Part model, mm, in its own coordinate system. Face numbers are marked on the shaded views. A direction names the side the tool comes from. Coordinates: 2 decimals unless noted, no trailing zeros. Loops run counter-clockwise (first coordinate to the right, second up) from the corner with the lowest first, then second, coordinate; pieces in that order, holes last. Notation, with made-up numbers: (-33, 67.5) - (23, 67.5) arc R19 cw to (23, 92.5) - close; hole circle Ø7 at (42.5, -9.5). An arc over 180 degrees is marked (long way). Use a Markdown table: item, result. Add a question column.
1. Drop flat-ended pins along their axis: pin 1 (5.5 mm diameter, centred on y = 8.5, z = -5, fed in from +X); pin 2 (9 mm diameter, centred on y = 9.5, z = 9.5, fed in from -X); pin 3 (4.5 mm diameter, centred on y = 19.3, z = 19.3, fed in from +X). Give the stop position or say it passes through.
2. 3-axis set-ups, long thin cutter, end or side, ignore diameter. For the marked faces 5 and 6: which of +Z, -Z, +X, -X, +Y, -Y reach the whole face in a straight line?
3. Band-saw the part on B-B, the plane z = 13.5. Give the cut face in (x, y), plus the area to 3 significant figures.
4. Band-saw the part on D-D, the plane y = -16. Give the cut face in (x, z), plus the area to 3 significant figures.
5. Wall check: probe 1 along Z at (x, y) = (6.5, -19.3) (3 decimals); probe 2 along Y at (x, z) = (33.5, -7); probe 3 along Y at (x, z) = (33, 13.5). Give the ranges that are in metal, low to high. Write a range as [from, to].
6. Pull direction Z, two halves, no side cores. Call the marked faces 1, 2, 3 and 4: pulls with the +Z half, pulls with the -Z half, needs draft (parallel to the pull), parting line crosses it, or undercut.
7. Band-saw the part on C-C, the plane y = -8. Give the cut face in (x, z), plus the area to 3 significant figures.
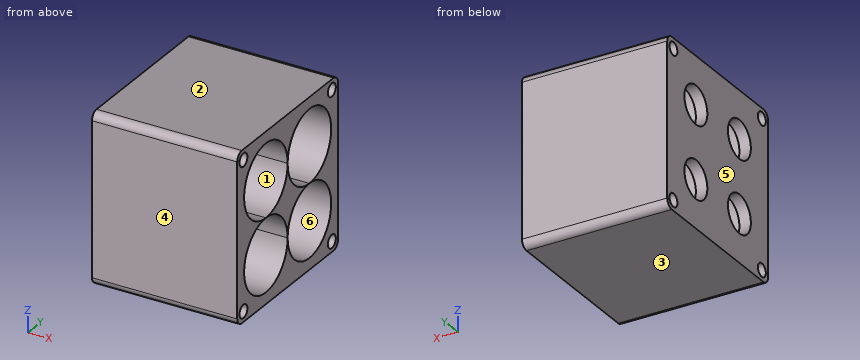
Autodesk Inventor part; units mm, degrees
ref_plane "YZ Plane" through (0, 0, 0) normal (1, 0, 0) x (0, 1, 0)
ref_plane "XZ Plane" through (0, 0, 0) normal (0, 1, 0) x (-1, 0, 0)
ref_plane "XY Plane" through (0, 0, 0) normal (0, 0, 1) x (1, 0, 0)
sketch "Sketch1" plane through (0, 0, 0) normal (1, 0, 0) x (0, 1, 0)
  line L0 (-22, -22) -> (22, -22)
  line L1 (22, -22) -> (22, 22)
  line L2 (22, 22) -> (-22, 22)
  line L3 (-22, 22) -> (-22, -22)
  line L4 (-22, -22) -> (22, 22) construction
  line L5 (22, -22) -> (-22, 22) construction
  line L6 (-19.3, -19.3) -> (19.3, -19.3)
  line L7 (19.3, -19.3) -> (19.3, 19.3)
  line L8 (19.3, 19.3) -> (-19.3, 19.3)
  line L9 (-19.3, 19.3) -> (-19.3, -19.3)
  line L10 (-19.3, -19.3) -> (19.3, 19.3) construction
  line L11 (19.3, -19.3) -> (-19.3, 19.3) construction
  circle A0 centre (19.3, 19.3) radius 1.725
  circle A1 centre (19.3, -19.3) radius 1.725
  circle A2 centre (-19.3, -19.3) radius 1.725
  circle A3 centre (-19.3, 19.3) radius 1.725
  circle A4 centre (9.5, 9.5) radius 9.5
  circle A5 centre (9.5, -9.5) radius 9.5
  circle A6 centre (-9.5, -9.5) radius 9.5
  circle A7 centre (-9.5, 9.5) radius 9.5
  point P0 (0, 0)
  point P1 (0, 0)
  point P2 (0, 0)
  point P3 (-9.5, 0)
  point P4 (0, 9.5)
  point P5 (9.5, 0)
  point P6 (0, -9.5)
  dimension "d4" = 44
  dimension "d5" = 44
  dimension "d6" = 38.6
  dimension "d7" = 3.45
  dimension "d8" = 3.45
  dimension "d9" = 3.45
  dimension "d10" = 3.45
  dimension "d24" = 19
  dimension "d25" = 19
  dimension "d26" = 19
  dimension "d27" = 19
extrude "Extrusion1" add sketch "Sketch1" along normal blind 35 contours L3 L2 L1 L0 | A2 L9 A3 L8 A0 L7 A1 L6 | A4 A5 A6 A7
fillet "Fillet1" radius 2 4 edges at (17.5, -22, 22) (17.5, -22, -22) (17.5, 22, 22) (17.5, 22, -22)
sketch "Sketch3" plane through (0, 0, 0) normal (-1, 0, 0) x (0, 0, 1)
  circle A0 centre (19.3, 19.3) radius 1.725
  arc A1 (0, -9.5) -> (9.5, 0) centre (9.5, -9.5) ccw
  arc A2 (-9.5, 0) -> (0, -9.5) centre (-9.5, -9.5) ccw
  arc A3 (0, 9.5) -> (-9.5, 0) centre (-9.5, 9.5) ccw
  arc A4 (9.5, 0) -> (0, 9.5) centre (9.5, 9.5) ccw
  circle A5 centre (-19.3, 19.3) radius 1.725
  circle A6 centre (-19.3, -19.3) radius 1.725
  circle A7 centre (19.3, -19.3) radius 1.725
  arc A8 (22, 20) -> (20, 22) centre (20, 20) ccw
  line L0 (-20, 22) -> (20, 22)
  line L1 (-22, -20) -> (-22, 20)
  arc A9 (-22, -20) -> (-20, -22) centre (-20, -20) ccw
  line L2 (20, -22) -> (-20, -22)
  arc A10 (20, -22) -> (22, -20) centre (20, -20) ccw
  line L3 (22, 20) -> (22, -20)
  circle A11 centre (9.5, -9.5) radius 5
  circle A12 centre (-9.5, -9.5) radius 5
  circle A13 centre (-9.5, 9.5) radius 5
  circle A14 centre (9.5, 9.5) radius 5
  arc A15 (-20, 22) -> (-22, 20) centre (-20, 20) ccw
  point P0 (0, 0)
  dimension "d28" = 10
  dimension "d29" = 10
  dimension "d30" = 10
  dimension "d31" = 10
extrude "Extrusion3" add sketch "Sketch3" along normal blind 3 contours A2 A3 A4 A1 | L3 A10 L2 A9 L1 A15 L0 A8
properties part number "BatteryHolder" material "ABS Plastic"
Geometry check:
| question | item | result |
|---|---|---|
| 1 | pin 1 | stops at x = 0 |
| 1 | pin 2 | passes through |
| 1 | pin 3 | stops at x = 35 |
| 2 | face 5 | +Z, -Z, -X, +Y, -Y |
| 2 | face 6 | +X |
| 3 | outline | (-3, -22) - (35, -22) - (35, -18.12) - (0, -18.12) - (0, -12.5) - (-3, -12.5) - close; (-3, -6.5) - (0, -6.5) - (0, -0.88) - (35, -0.88) - (35, 0.88) - (0, 0.88) - (0, 6.5) - (-3, 6.5) - close; (-3, 12.5) - (0, 12.5) - (0, 18.12) - (35, 18.12) - (35, 22) - (-3, 22) - close |
| 3 | area | 430 mm^2 |
| 4 | outline | (-3, -22) - (35, -22) - (35, -16.43) - (0, -16.43) - (0, -2.57) - (35, -2.57) - (35, 2.57) - (0, 2.57) - (0, 16.43) - (35, 16.43) - (35, 22) - (-3, 22) - close |
| 4 | area | 702 mm^2 |
| 5 | probe 1 | z = [-22, -21.025], [-17.575, 17.575], [21.025, 22] |
| 5 | probe 2 | y = [-22, -18.67], [-0.33, 0.33], [18.67, 22] |
| 5 | probe 3 | y = [-22, -18.12], [-0.88, 0.88], [18.12, 22] |
| 6 | face 1 | undercut |
| 6 | face 2 | pulls with the +Z half |
| 6 | face 3 | pulls with the -Z half |
| 6 | face 4 | needs draft |
| 7 | outline | (-3, -22) - (35, -22) - (35, -18.88) - (0, -18.88) - (0, -14.27) - (-3, -14.27) - close; (-3, -4.73) - (0, -4.73) - (0, -0.12) - (35, -0.12) - (35, 0.12) - (0, 0.12) - (0, 4.73) - (-3, 4.73) - close; (-3, 14.27) - (0, 14.27) - (0, 18.88) - (35, 18.88) - (35, 22) - (-3, 22) - close |
| 7 | area | 301 mm^2 |
